Can you work these out from the model? Positions are in its coordinate system, mm. A direction names the side the tool comes from. Round coordinates to 2 decimals unless told otherwise and drop trailing zeros. Order: outer loops, then holes, each group sorted by start corner. A loop starts at its lowest first (then second) coordinate and runs counter-clockwise, first axis right, second up.
Q1. If we section it at C-C (z = 1.25): Please give me the cut outline in (x, y), plus the area to 3 significant figures.
Q2. We'd pull the mould along Z, two halves only. Please class faces 1 (the face through (24, 1, 0)), 2 (the face through (0.45, 1.48, 1.43)), 3 (the face through (8, 3, 0)), 4 (the face through (15.323, 1.521, -2.243)): pulls with the +Z half, pulls with the -Z half, needs draft (parallel to the pull), parting line crosses it, or undercut.
Q3. Will these pins go through, and if not, where does the flat tip stop? P1, Ø1.5, axis at x = 21.5, y = 2, coming from the -Z side; P2, Ø2.5, axis at x = 25, z = 0, coming from the -Y side; P3, Ø1, axis at x = 17.5, y = 1, coming from the +Z side.
Q4. If we section it at B-B (y = 2.2): Please give me the cut outline in (x, z), plus the area to 3 significant figures.
Q5. If we section it at D-D (x = 21.75): Please give me the cut outline in (y, z), plus the area to 3 significant figures.
Q6. For faces 5 (the face through (23, 1, -2)), 6 (the face through (8.536, 1.479, -0.325)), 7 (the face through (23, 1, 2)), which set-ups out of +Z, -Z, +X, -X, +Y, -Y let a thin tool reach every point of the face, with its end or its side?
Q7. If I drill on line 1 (X direction, y = 1.45, z = 0); line 2 (X direction, y = 0.35, z = 1.05); line 3 (X direction, y = 0.65, z = -0.5), over which ranges is the centre line in solid material (lowest first)?
Q8. If we section it at A-A (z = 0): Please give me the cut outline in (x, y).
from build123d import *

# Parameters (mm, degrees)
SKETCH1_R           = 1
SKETCH1_R_2         = 1.5
BOSS_EXTRUDE1_DEPTH = 3
FILLET1_R           = 50


with BuildPart() as part:
    # Sketch1 → Boss-Extrude1 (new body)
    # profile 1 of 3: a face of its own
    with BuildSketch(Plane(origin=(0, 0, 0), x_dir=(1, 0, 0), z_dir=(0, 1, 0))):
        with BuildLine():
            Line((25, 2), (12.236067977, 2))
            ThreePointArc((12.236067977, 2), (13, 0), (12.236067977, -2))
            Line((12.236067977, -2), (25, -2))
            ThreePointArc((25, -2), (27, 0), (25, 2))
        make_face()
        with Locations(Location((25, 0, 0), (0, 0, 270))):
            Circle(SKETCH1_R, mode=Mode.SUBTRACT)
    # profile 2 of 3: a face of its own
    with BuildSketch(Plane(origin=(0, 0, 0), x_dir=(1, 0, 0), z_dir=(0, 1, 0))):
        with BuildLine():
            ThreePointArc((12.236067977, -2), (13, 0), (12.236067977, 2))
            Line((12.236067977, 2), (10, 2))
            ThreePointArc((10, 2), (8, 0), (10, -2))
            Line((10, -2), (12.236067977, -2))
        make_face()
        with Locations(Location((10, 0, 0), (0, 0, 270))):
            Circle(SKETCH1_R_2, mode=Mode.SUBTRACT)
    # profile 3 of 3: a face of its own
    with BuildSketch(Plane(origin=(0, 0, 0), x_dir=(1, 0, 0), z_dir=(0, 1, 0))):
        with BuildLine():
            Line((10, 3), (0, 3))
            ThreePointArc((0, 3), (-3, 0), (0, -3))
            Line((0, -3), (10, -3))
            ThreePointArc((10, -3), (11.224744871, -2.738612788), (12.236067977, -2))
            Line((12.236067977, -2), (10, -2))
            ThreePointArc((10, -2), (8, 0), (10, 2))
            Line((10, 2), (12.236067977, 2))
            ThreePointArc((12.236067977, 2), (11.224744871, 2.738612788), (10, 3))
        make_face()
        with Locations(Location((0, 0, 0), (0, 0, 270))):
            Circle(SKETCH1_R_2, mode=Mode.SUBTRACT)
    extrude(amount=BOSS_EXTRUDE1_DEPTH)

    # Fillet1
    fillet1_edges = [part.edges().sort_by_distance(p)[0] for p in [
        (12.236067977, 1.5, 2),
        (12.236067977, 1.5, -2),
    ]]
    fillet(fillet1_edges, radius=FILLET1_R)


solid = part.part
Solution:
1. outline: (-2.73, 0) - (-0.83, 0) - (-0.83, 3) - (-2.73, 3) - close; (0.83, 0) - (9.17, 0) - (9.17, 3) - (0.83, 3) - close; (10.83, 0) - (26.56, 0) - (26.56, 3) - (10.83, 3) - close
1. area: 77.9 mm2
2. face 1: undercut
2. face 2: undercut
2. face 3: needs draft
2. face 4: pulls with the -Z half
3. P1: stops at z = -2
3. P2: stops at y = 0
3. P3: stops at z = 2.11
4. outline: (0, -3) - (10, -3) arc R3 ccw to (10.58, -2.94) arc R50 cw to (20.25, -2) - (25, -2) arc R2 ccw to (25, 2) - (20.25, 2) arc R50 cw to (10.58, 2.94) arc R3 ccw to (10, 3) - (0, 3) arc R3 ccw to start; hole circle Ø3 at (0, 0); hole circle Ø3 at (10, 0); hole circle Ø2 at (25, 0)
4. area: 130 mm2
5. outline: (0, -2) - (3, -2) - (3, 2) - (0, 2) - close
5. area: 12.0 mm2
6. face 5: -Z, +X, +Y, -Y
6. face 6: +Y, -Y
6. face 7: +Z, +X, +Y, -Y
7. line 1: x = -3 to -1.5, 1.5 to 8.5, 11.5 to 24, 26 to 27
7. line 2: x = -2.81 to -1.07, 1.07 to 8.93, 11.07 to 26.7
7. line 3: x = -2.96 to -1.41, 1.41 to 8.59, 11.41 to 24.13, 25.87 to 26.94
8. outline: (-3, 0) - (-1.5, 0) - (-1.5, 3) - (-3, 3) - close; (1.5, 0) - (8.5, 0) - (8.5, 3) - (1.5, 3) - close; (11.5, 0) - (24, 0) - (24, 3) - (11.5, 3) - close; (26, 0) - (27, 0) - (27, 3) - (26, 3) - close
